```python
from build123d import *

# Parameters (mm, degrees)
SKETCH1_W                   = 205.74
SKETCH1_H                   = 33.02
SKETCH1_W_2                 = 201.74
SKETCH1_H_2                 = 29.02
SKETCH1_R                   = 3.175
BOSS_EXTRUDE1_DEPTH         = 4.5
TAP_DRILL_FOR_M3X0_5_TAP1_D = 2.5
SKETCH5_W                   = 235.74
SKETCH5_H                   = 35.94
BOSS_EXTRUDE2_DEPTH         = 2
SKETCH6_W                   = 53.1
SKETCH6_H                   = 2.92
BOSS_EXTRUDE3_DEPTH         = 5.65
F_1_4_CLEARANCE_HOLE1_D     = 6.7564


with BuildPart() as part:
    # Sketch1 → Boss-Extrude1 (new body)
    # profile 1 of 6: a face of its own
    with BuildSketch(Plane(origin=(0, 0, 143.199899198), x_dir=(-1, 0, 0), z_dir=(0, 0, -1))):
        with Locations((-78.001678372, 116.22318568)):
            Rectangle(SKETCH1_W, SKETCH1_H)
        with Locations((-78.001678372, 116.22318568)):
            Rectangle(SKETCH1_W_2, SKETCH1_H_2, mode=Mode.SUBTRACT)
    # profile 2 of 6: a face of its own
    with BuildSketch(Plane(origin=(0, 0, 143.199899198), x_dir=(-1, 0, 0), z_dir=(0, 0, -1))):
        with BuildLine():
            Line((16.518321628, 107.06318568), (16.518321628, 101.71318568))
            Line((16.518321628, 101.71318568), (22.868321628, 101.71318568))
            Line((22.868321628, 101.71318568), (22.868321628, 108.06318568))
            Line((22.868321628, 108.06318568), (17.518321628, 108.06318568))
            ThreePointArc((17.518321628, 108.06318568), (16.811214846, 107.770292461), (16.518321628, 107.06318568))
        make_face()
    # profile 3 of 6: a face of its own
    with BuildSketch(Plane(origin=(0, 0, 143.199899198), x_dir=(-1, 0, 0), z_dir=(0, 0, -1))):
        with BuildLine():
            Line((22.868321628, 130.73318568), (16.518321628, 130.73318568))
            Line((16.518321628, 130.73318568), (16.518321628, 125.38318568))
            ThreePointArc((16.518321628, 125.38318568), (16.811214846, 124.676078899), (17.518321628, 124.38318568))
            Line((17.518321628, 124.38318568), (22.868321628, 124.38318568))
            Line((22.868321628, 124.38318568), (22.868321628, 130.73318568))
        make_face()
    # profile 4 of 6: a face of its own
    with BuildSketch(Plane(origin=(0, 0, 143.199899198), x_dir=(-1, 0, 0), z_dir=(0, 0, -1))):
        with Locations((-118.641678372, 121.30318568)):
            Circle(SKETCH1_R)
    # profile 5 of 6: a face of its own
    with BuildSketch(Plane(origin=(0, 0, 143.199899198), x_dir=(-1, 0, 0), z_dir=(0, 0, -1))):
        with BuildLine():
            Line((-178.871678372, 130.73318568), (-178.871678372, 124.38318568))
            Line((-178.871678372, 124.38318568), (-173.521678372, 124.38318568))
            ThreePointArc((-173.521678372, 124.38318568), (-172.814571591, 124.676078899), (-172.521678372, 125.38318568))
            Line((-172.521678372, 125.38318568), (-172.521678372, 130.73318568))
            Line((-172.521678372, 130.73318568), (-178.871678372, 130.73318568))
        make_face()
    # profile 6 of 6: a face of its own
    with BuildSketch(Plane(origin=(0, 0, 143.199899198), x_dir=(-1, 0, 0), z_dir=(0, 0, -1))):
        with BuildLine():
            Line((-178.871678372, 108.06318568), (-178.871678372, 101.71318568))
            Line((-178.871678372, 101.71318568), (-172.521678372, 101.71318568))
            Line((-172.521678372, 101.71318568), (-172.521678372, 107.06318568))
            ThreePointArc((-172.521678372, 107.06318568), (-172.814571591, 107.770292461), (-173.521678372, 108.06318568))
            Line((-173.521678372, 108.06318568), (-178.871678372, 108.06318568))
        make_face()
    extrude(amount=BOSS_EXTRUDE1_DEPTH)

    # Tap Drill for M3x0.5 Tap1 (through all)
    with Locations(Plane.XY.offset(143.199899198)):
        with Locations((-19.788321628, 127.65318568), (-19.788321628, 104.79318568), (118.641678372, 121.30318568), (175.791678372, 127.65318568), (175.791678372, 104.79318568)):
            Hole(TAP_DRILL_FOR_M3X0_5_TAP1_D / 2)

    # Sketch5 → Boss-Extrude2 (add)
    with BuildSketch(Plane(origin=(0, 0, 138.699899198), x_dir=(-1, 0, 0), z_dir=(0, 0, -1))):
        with Locations((-78.001678372, 117.68318568)):
            Rectangle(SKETCH5_W, SKETCH5_H)
    extrude(amount=BOSS_EXTRUDE2_DEPTH)

    # Sketch6 → Boss-Extrude3 (add)
    with BuildSketch(Plane.XY.offset(138.699899198)):
        with Locations((84.241678372, 134.19318568)):
            Rectangle(SKETCH6_W, SKETCH6_H)
    extrude(amount=BOSS_EXTRUDE3_DEPTH)

    # 1/4 Clearance Hole1 (through all)
    with Locations(Plane.XY.offset(138.699899198)):
        with Locations((190.871678372, 104.98318568), (190.871678372, 130.38318568), (-34.868321628, 104.98318568), (-34.868321628, 130.38318568)):
            Hole(F_1_4_CLEARANCE_HOLE1_D / 2)


solid = part.part
```
For this review, take the finished solid that the model builds, in its own axes (mm). A direction names the side the tool comes from. Round coordinates to 2 decimals unless told otherwise and drop trailing zeros. Write each loop counter-clockwise with the first axis right and the second up, starting at its lowest first coordinate (ties: lowest second). Pieces come first, ordered by that corner, then holes.
1) Machinability: for faces 4 (the face through (-20, 108.063, 141)), 5 (the face through (-24.868, 116, 141)), 6 (the face through (-32.187, 128.328, 137.686)), 7 (the face through (86, 131, 143.2)), which of the approach directions +Z, -Z, +X, -X, +Y, -Y give a long, thin tool a straight path to every point of the face, cutting with its end or side? Answer none if there is none.
Answer below:
face 4: +Z
face 5: +Z, -X, +Y, -Y
face 6: +Z, -Z
face 7: +Z, +X, -X, -Y
2) Take a section at A-A on z = 141. State how many separate pieces and enclosed holes the cut face has, then the cut area to 3 significant figures.
Answer below:
separate pieces: 2
enclosed holes: 6
area: 1,260 mm2
3) For line 1 along X through (y, z) = (105, 138.25); line 2 along Y through (x, z) = (2.5, 141.75); line 3 along X through (y, z) = (128, 143), list the stretches that pass through material, from the lowest coordinate up.
Answer below:
line 1: x = -39.87 to -38.25, -31.49 to 187.49, 194.25 to 195.87
line 2: y = 99.71 to 101.71, 130.73 to 132.73
line 3: x = -24.87 to -20.99, -18.59 to -16.52, 172.52 to 174.59, 176.99 to 180.87
4) Mouldability with a two-part tool opening along Y and no side actions: class faces 1 (the face through (79, 116, 138.7)), 2 (the face through (146, 132.733, 141)), 3 (the face through (-16, 134, 138.7)) as +Y half, -Y half, draft (parallel to the pull), parting line (faces both ways), or undercut.
Answer below:
face 1: undercut
face 2: +Y half
face 3: draft
5) Take a section at C-C on y = 110.5. Give the boundary of the cut face in (x, z), then the cut area to 3 significant figures.
Answer below:
outline: (-39.87, 136.7) - (195.87, 136.7) - (195.87, 138.7) - (180.87, 138.7) - (180.87, 143.2) - (178.87, 143.2) - (178.87, 138.7) - (-22.87, 138.7) - (-22.87, 143.2) - (-24.87, 143.2) - (-24.87, 138.7) - (-39.87, 138.7) - close
area: 489 mm2
6) Insertion check: pin 1 Ø1.5 at (x, y) = (118.64, 121.3) entering from +Z; pin 2 Ø2 at (x, z) = (118, 140) entering from +Y; pin 3 Ø3 at (x, y) = (118, 121.5) entering from +Z; pin 4 Ø6 at (x, y) = (-34.87, 130.38) entering from -Z. Each pin has a flat end and moves straight along its axis. Give the tip position at first contact, or say it passes through.
Answer below:
pin 1: stops at z = 138.7
pin 2: stops at y = 132.73
pin 3: stops at z = 143.2
pin 4: passes through
7) Take a section at D-D on x = 75.5. Give the boundary of the cut face in (y, z).
Answer below:
outline: (99.71, 136.7) - (135.65, 136.7) - (135.65, 144.35) - (132.73, 144.35) - (132.73, 143.2) - (130.73, 143.2) - (130.73, 138.7) - (101.71, 138.7) - (101.71, 143.2) - (99.71, 143.2) - close
8) Take a section at B-B on x = -0.5. Give the boundary of the cut face in (y, z), then the cut area to 3 significant figures.
Answer below:
outline: (99.71, 136.7) - (135.65, 136.7) - (135.65, 138.7) - (132.73, 138.7) - (132.73, 143.2) - (130.73, 143.2) - (130.73, 138.7) - (101.71, 138.7) - (101.71, 143.2) - (99.71, 143.2) - close
area: 89.9 mm2
